Can you work these out from the drawing? Everything is in mm from the part's minimum corner. A direction names the side the tool comes from. Coordinates: 2 decimals unless noted, no trailing zeros. Loops run counter-clockwise (first coordinate to the right, second up) from the corner with the lowest first, then second, coordinate; pieces in that order, holes last. Notation, with made-up numbers: (36.25, 81.5) -> (58.25, 81.5) arc R27 cw to (58.25, 108.5) -> close; hole circle Ø9 at (53.25, -17). An arc over 180 degrees is marked (long way). Use one line per item in the form item = value. Start each with the question number.
(1) Imagine slicing it at A-A (z = 5.9). List the corners of the cut face in (x, y) for me.
(2) Imagine slicing it at B-B (x = 6.5). List the corners of the cut face in (y, z) for me.
(3) I'm going to push flat-ended pins straight in: pin 1 (5 mm diameter, centred on x = 22.5, z = 9.5, fed in from +Y); pin 2 (3.5 mm diameter, centred on y = 21, z = 7, fed in from -X); pin 3 (1.5 mm diameter, centred on x = 17.5, z = 3.5, fed in from -Y); pin 4 (6 mm diameter, centred on y = 7, z = 6.5, fed in from +X). Where does each tip first touch, or does it pass through?
(4) On a 3-axis mill with a long thin cutter (end or side, diameter ignored), from which of +Z, -Z, +X, -X, +Y, -Y can I reach the whole of each face in a straight line? I mean the marked faces 1, 2 and 3. Say none if no direction works.
(5) I need wall thicknesses on line 1 (Y direction, x = 17, z = 7); line 2 (X direction, y = 5, z = 8.75); line 3 (Y direction, x = 29.5, z = 7). Which ranges of each line are inside material? Lowest first, please. Write a range as [from, to].
(6) Imagine slicing it at C-C (y = 4.25). List the corners of the cut face in (x, z) for me.
(7) Imagine slicing it at D-D (z = 3). List the corners of the cut face in (x, y) for me (1 decimal), plus the area to 3 significant figures.
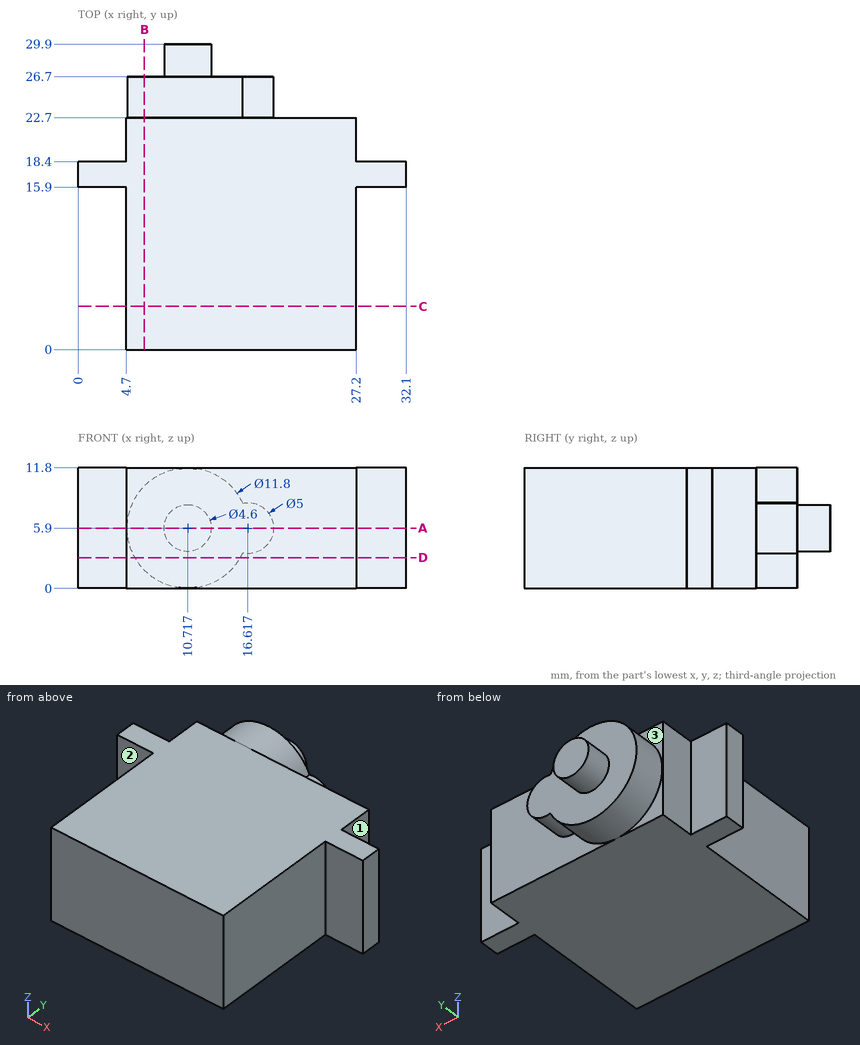
Worked out:
q1.outline = (0, 15.9) -> (4.7, 15.9) -> (4.7, 0) -> (27.2, 0) -> (27.2, 15.9) -> (32.1, 15.9) -> (32.1, 18.4) -> (27.2, 18.4) -> (27.2, 22.7) -> (19.12, 22.7) -> (19.12, 26.7) -> (13.02, 26.7) -> (13.02, 29.9) -> (8.42, 29.9) -> (8.42, 26.7) -> (4.82, 26.7) -> (4.82, 22.7) -> (4.7, 22.7) -> (4.7, 18.4) -> (0, 18.4) -> close
q2.outline = (0, 0) -> (22.7, 0) -> (22.7, 1.77) -> (26.7, 1.77) -> (26.7, 10.03) -> (22.7, 10.03) -> (22.7, 11.8) -> (0, 11.8) -> close
q3.pin_1 = 22.7
q3.pin_2 = 4.7
q3.pin_3 = 0
q3.pin_4 = 27.2
q4.face_1 = +Z, -Z, +X, +Y
q4.face_2 = +Z, -Z, -X, -Y
q4.face_3 = -X, +Y
q5.line_1 = [0, 26.7]
q5.line_2 = [4.7, 27.2]
q5.line_3 = [15.9, 18.4]
q6.outline = (4.7, 0) -> (27.2, 0) -> (27.2, 11.8) -> (4.7, 11.8) -> close
q7.outline = (0, 15.9) -> (4.7, 15.9) -> (4.7, 0) -> (27.2, 0) -> (27.2, 15.9) -> (32.1, 15.9) -> (32.1, 18.4) -> (27.2, 18.4) -> (27.2, 22.7) -> (15.9, 22.7) -> (15.9, 26.7) -> (5.6, 26.7) -> (5.6, 22.7) -> (4.7, 22.7) -> (4.7, 18.4) -> (0, 18.4) -> close
q7.area = 576 mm2
